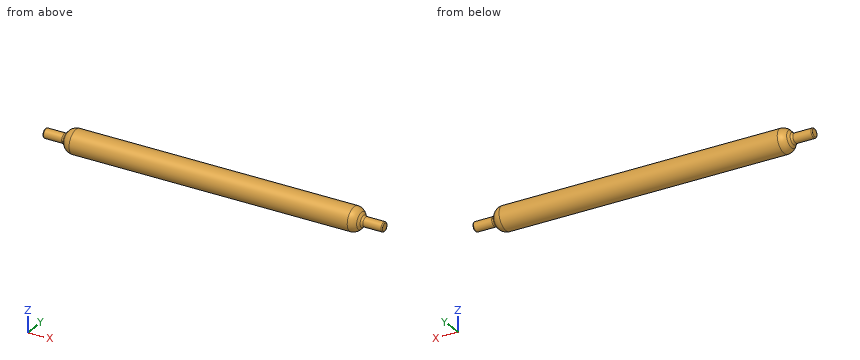
```python
from build123d import *


with BuildPart() as f1:
    # F0 (on Front) → F1 (revolve)
    with BuildSketch(Plane.XZ):
        with BuildLine():
            Line((0, 8), (0, 0))
            Line((0, 0), (360, 0))
            Line((360, 0), (720, 0))
            Line((720, 0), (720, 8))
            ThreePointArc((720, 8), (719.414214, 9.414214), (718, 10))
            Line((718, 10), (679.542538, 10))
            ThreePointArc((679.542538, 10), (677.031904, 10.571547), (675.016079, 12.173546))
            Line((675.016079, 12.173546), (670.744676, 17.505015))
            ThreePointArc((670.744676, 17.505015), (663.793556, 23.029147), (655.136198, 25))
            Line((655.136198, 25), (360, 25))
            Line((360, 25), (64.863802, 25))
            ThreePointArc((64.863802, 25), (56.206444, 23.029147), (49.255324, 17.505015))
            Line((49.255324, 17.505015), (44.983921, 12.173546))
            ThreePointArc((44.983921, 12.173546), (42.968096, 10.571547), (40.457462, 10))
            Line((40.457462, 10), (2, 10))
            ThreePointArc((2, 10), (0.585786, 9.414214), (0, 8))
        make_face()
    revolve(axis=Axis((180, 0, 0), (1, 0, 0)))


solid = f1.part
```
Verification items for the finished model (mm, model axes). Give positions to 0.01 mm unless a question says otherwise; leave off trailing zeros. Order: outer loops, then holes, each group sorted by start corner. A loop starts at its lowest first (then second) coordinate and runs counter-clockwise, first axis right, second up. Notation, with made-up numbers: (76, -20) -> (103, -20) arc R21 ccw to (103, 1) -> close; hole circle Ø2 at (34, 38.25). An arc over 180 degrees is marked (long way). One line per item, written item: value.
(1) Scan lines: line 1 along Y through (x, z) = (257, 1); line 2 along Z through (x, y) = (644, 1.5); line 3 along Z through (x, y) = (416.5, -16.5). Record each from-to range of solid material in increasing order. Write a range as [from, to].
Final values:
line 1: [-24.98, 24.98]
line 2: [-24.95, 24.95]
line 3: [-18.78, 18.78]
(2) Sectioned sample at A-A on x = 287. Record the cut outline in (y, z), then the cut area to 3 significant figures.
Final values:
outline: circle Ø50 at (0, 0)
area: 1,960 mm^2
(3) Gauge pin test, flat ends, axial feed: pin 1 (3 mm diameter, centred on y = 17, z = 5.5, fed in from +X); pin 2 (1 mm diameter, centred on y = 18, z = 1, fed in from -X); pin 3 (10 mm diameter, centred on y = -17, z = 13, fed in from +X). Record the tip position at first contact, or that the pin passes through.
Final values:
pin 1: x = 671.66
pin 2: x = 49.27
pin 3: x = 671.63
